Geometry check sheet. Reference: the model listing, model coordinates, mm. Face numbers are marked on the shaded views. A direction names the side the tool comes from. Round coordinates to 2 decimals unless told otherwise and drop trailing zeros. Order: outer loops, then holes, each group sorted by start corner. A loop starts at its lowest first (then second) coordinate and runs counter-clockwise, first axis right, second up.
(1) Material ranges on line 1 along Z through (x, y) = (4.75, 5.25); line 2 along Z through (x, y) = (3.5, 8.5) (3 decimals); line 3 along X through (y, z) = (1.5, -4.5), recorded low to high.
(2) Sectioned sample at B-B (x = -5.75). Give the number of separate pieces and of enclosed holes in the cut face, plus the area to 3 significant figures.
(3) Go/stop test with flat-tipped pins: pin 1 (5 mm diameter, centred on x = -7, y = 6.5, fed in from +Z); pin 2 (1 mm diameter, centred on y = 1.5, z = 8.5, fed in from +X); pin 3 (1.2 mm diameter, centred on y = 7, z = 4, fed in from -X). Record where each tip stops, or that it passes through.
(4) Sectioned sample at A-A (y = 7.5). Record the boundary of the cut face in (x, z) (1 decimal), plus the area to 3 significant figures.
(5) Sectioned sample at D-D (y = 3). Record the boundary of the cut face in (x, z) (1 decimal), plus the area to 3 significant figures.
(6) Release check for a two-part mould opening along Z. For the marked faces 3, 4 and 5 record: +Z half, -Z half, draft (parallel to the pull), parting line (faces both ways), or undercut.
(7) Set-up check for the marked faces 1 and 2: record each of +Z, -Z, +X, -X, +Y, -Y from which the full face is reachable in a straight line by a thin tool's end or side.
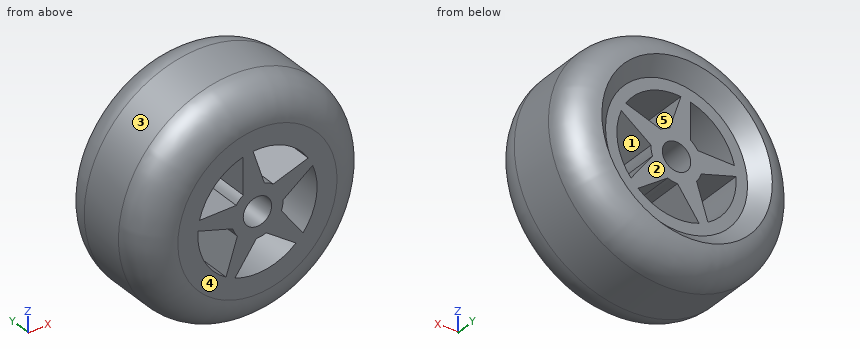
from build123d import *

# Parameters (mm, degrees)
F3_R     = 1.5875
F4_DEPTH = 12.7
F6_DEPTH = 25.4


# Not quite as in the source:
# - a fillet or chamfer that OpenCascade refuses, or shapes differently, is made with other operations: its cross-section is extruded or revolved along the edge and cut away or added


with BuildPart() as f1:
    # F0 (on Right) → F1 (revolve)
    with BuildSketch(Plane.YZ):
        Polygon((0, 12.7), (0, 0), (11.1125, 0), (11.1125, 7.9375), (12.7, 9.525), (12.7, 12.7), align=None)
    revolve(axis=Axis((0, 5.55625, 0), (0, -1, 0)))

    # F2: fillet of radius 3.81 on 2 edges, made by hand

    # F2_s1 → F2_t2 (revolve, cut)
    with BuildSketch(Plane.YZ):
        with BuildLine():
            ThreePointArc((0, 8.89), (1.1159231637, 11.5840768363), (3.81, 12.7))
            Line((3.81, 12.7), (0, 12.7))
            Line((0, 12.7), (0, 8.89))
        make_face()
    revolve(axis=Axis((0, 0, 0), (0, -1, 0)), mode=Mode.SUBTRACT)

    # F2_s3 → F2_t4 (revolve, cut)
    with BuildSketch(Plane.YZ):
        with BuildLine():
            ThreePointArc((12.7, 9.525), (11.4026337626, 11.7999355663), (8.9432893377, 12.7))
            Line((8.9432893377, 12.7), (12.7, 12.7))
            Line((12.7, 12.7), (12.7, 9.525))
        make_face()
    revolve(axis=Axis((0, 12.7, 0), (0, -1, 0)), mode=Mode.SUBTRACT)

    # F3 (on face) → F4 (cut)
    with BuildSketch(Plane(origin=(0, 11.1125, 0), x_dir=(-1, 0, 0), z_dir=(0, 1, 0))):
        Circle(F3_R)
    extrude(amount=-F4_DEPTH, mode=Mode.SUBTRACT)

    # F5 (on face) → F6 (cut)
    with BuildSketch(Plane(origin=(0, 11.1125, 0), x_dir=(-1, 0, 0), z_dir=(0, 1, 0))):
        with BuildLine():
            Line((-5.668244305, 3.5109204987), (-1.7691005725, 2.2440119016))
            ThreePointArc((-1.7691005725, 2.2440119016), (-1.297277853, 2.5460511429), (-0.7755925376, 2.7502295296))
            Line((-0.7755925376, 2.7502295296), (0.4913160595, 6.6493732622))
            ThreePointArc((0.4913160595, 6.6493732622), (-3.026981657, 5.940786), (-5.668244305, 3.5109204987))
        make_face()
        with BuildLine():
            ThreePointArc((1.5875, 2.3759524406), (2.0205576272, 2.0205576272), (2.3759524406, 1.5875))
            Line((2.3759524406, 1.5875), (6.4757547823, 1.5875))
            ThreePointArc((6.4757547823, 1.5875), (4.7146344636, 4.7146344636), (1.5875, 6.4757547823))
            Line((1.5875, 6.4757547823), (1.5875, 2.3759524406))
        make_face()
        with BuildLine():
            Line((-5.090667637, -4.3058865822), (-2.6808642833, -0.9890768143))
            ThreePointArc((-2.6808642833, -0.9890768143), (-2.8223194333, -0.4470114839), (-2.8552949903, 0.1122353262))
            Line((-2.8552949903, 0.1122353262), (-6.1721047583, 2.5220386799))
            ThreePointArc((-6.1721047583, 2.5220386799), (-6.5854120109, -1.0430267957), (-5.090667637, -4.3058865822))
        make_face()
        with BuildLine():
            Line((2.5220386799, -6.1721047583), (0.1122353262, -2.8552949903))
            ThreePointArc((0.1122353262, -2.8552949903), (-0.4470114839, -2.8223194333), (-0.9890768143, -2.6808642833))
            Line((-0.9890768143, -2.6808642833), (-4.3058865822, -5.090667637))
            ThreePointArc((-4.3058865822, -5.090667637), (-1.0430267957, -6.5854120109), (2.5220386799, -6.1721047583))
        make_face()
        with BuildLine():
            Line((6.6493732622, 0.4913160595), (2.7502295296, -0.7755925376))
            ThreePointArc((2.7502295296, -0.7755925376), (2.5460511429, -1.297277853), (2.2440119016, -1.7691005725))
            Line((2.2440119016, -1.7691005725), (3.5109204987, -5.668244305))
            ThreePointArc((3.5109204987, -5.668244305), (5.940786, -3.026981657), (6.6493732622, 0.4913160595))
        make_face()
    extrude(amount=-F6_DEPTH, mode=Mode.SUBTRACT)


solid = f1.part
Answer below:
1. line 1: z = -11.78 to -3.84, 1.49 to 3.21, 4.68 to 11.78
1. line 2: z = -12.208 to -5.675, -4.505 to -2.117, 0.581 to 2.806, 5.675 to 12.208
1. line 3: x = -11.04 to -4.92, -3.13 to -1.31, 3.49 to 11.04
2. separate pieces: 3
2. enclosed holes: 0
2. area: 193 mm2
3. pin 1: stops at z = 11.88
3. pin 2: stops at x = 9.03
3. pin 3: stops at x = -12.24
4. outline: circle Ø25.4 at (0, 0); hole (-6.6, 0.5) arc R6.7 ccw to (-3.5, -5.7) - (-2.2, -1.8) arc R2.9 cw to (-2.8, -0.8) - close; hole (-6.5, 1.6) - (-2.4, 1.6) arc R2.9 cw to (-1.6, 2.4) - (-1.6, 6.5) arc R6.7 ccw to start; hole (-2.5, -6.2) arc R6.7 ccw to (4.3, -5.1) - (1, -2.7) arc R2.9 cw to (-0.1, -2.9) - close; hole circle Ø3.2 at (0, 0); hole (-0.5, 6.6) - (0.8, 2.8) arc R2.9 cw to (1.8, 2.2) - (5.7, 3.5) arc R6.7 ccw to start; hole (2.7, -1) - (5.1, -4.3) arc R6.7 ccw to (6.2, 2.5) - (2.9, 0.1) arc R2.9 cw to start
4. area: 418 mm2
5. outline: circle Ø25.2 at (0, 0); hole (-6.6, 0.5) arc R6.7 ccw to (-3.5, -5.7) - (-2.2, -1.8) arc R2.9 cw to (-2.8, -0.8) - close; hole (-6.5, 1.6) - (-2.4, 1.6) arc R2.9 cw to (-1.6, 2.4) - (-1.6, 6.5) arc R6.7 ccw to start; hole (-2.5, -6.2) arc R6.7 ccw to (4.3, -5.1) - (1, -2.7) arc R2.9 cw to (-0.1, -2.9) - close; hole circle Ø3.2 at (0, 0); hole (-0.5, 6.6) - (0.8, 2.8) arc R2.9 cw to (1.8, 2.2) - (5.7, 3.5) arc R6.7 ccw to start; hole (2.7, -1) - (5.1, -4.3) arc R6.7 ccw to (6.2, 2.5) - (2.9, 0.1) arc R2.9 cw to start
5. area: 411 mm2
6. face 3: parting line
6. face 4: draft
6. face 5: undercut
7. face 1: +Y, -Y
7. face 2: +Y
